from build123d import *

# Parameters (mm, degrees)
SKETCH_1_R          = 7
EXTRUDE_1_DEPTH     = 1
SKETCH_2_R          = 5
EXTRUDE_2_DEPTH     = 6
EXTRUDE_START       = 11
SKETCH_3_R          = 7
EXTRUDE_3_DEPTH     = 11
SKETCH_4_R          = 4
CUT_EXTRUDE_1_DEPTH = 21.542638584


with BuildPart() as part:
    # Эскиз1 → Бобышка-Вытянуть1 (new body)
    with BuildSketch(Plane.XY):
        Circle(SKETCH_1_R)
    extrude(amount=EXTRUDE_1_DEPTH)

    # Эскиз2 → Бобышка-Вытянуть2 (add)
    with BuildSketch(Plane(origin=(0, 0, 0), x_dir=(-1, 0, 0), z_dir=(0, 0, -1))):
        with Locations(Location((0, 0, 0), (0, 0, 180))):
            Circle(SKETCH_2_R)
    extrude(amount=EXTRUDE_2_DEPTH)

    # Эскиз3 → Бобышка-Вытянуть3 (add)
    with BuildSketch(Plane(origin=(0, 0, -6), x_dir=(-1, 0, 0), z_dir=(0, 0, -1)).offset(EXTRUDE_START)):
        with Locations(Location((0, 0, 0), (0, 0, 180))):
            Circle(SKETCH_3_R)
    extrude(amount=-EXTRUDE_3_DEPTH)

    # Эскиз4 → Вырез-Вытянуть1 (cut, through all)
    with BuildSketch(Plane(origin=(0, 0, -17), x_dir=(-1, 0, 0), z_dir=(0, 0, -1))):
        Circle(SKETCH_4_R)
    extrude(amount=-CUT_EXTRUDE_1_DEPTH, mode=Mode.SUBTRACT)


solid = part.part
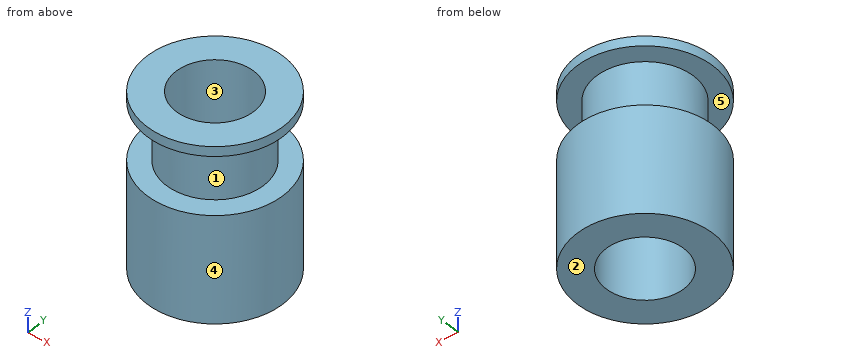
Verification items for the finished model (mm, model axes). Face numbers are marked on the shaded views. A direction names the side the tool comes from. Round coordinates to 2 decimals unless told otherwise and drop trailing zeros. Write each loop counter-clockwise with the first axis right and the second up, starting at its lowest first coordinate (ties: lowest second). Pieces come first, ordered by that corner, then holes.
(1) Mould release check, pull along Y, two halves, no side actions. Record for the marked faces 3, 4 and 5: pulls with the +Y half, pulls with the -Y half, needs draft (parallel to the pull), parting line crosses it, or undercut.
Returned:
face 3: undercut
face 4: parting line crosses it
face 5: needs draft
(2) Depth check by flat-ended pin: pin 1 Ø1 at (y, z) = (1, -4.5) entering from -X; pin 2 Ø4 at (x, z) = (4.5, -10.5) entering from +Y; pin 3 Ø8 at (x, z) = (-5.5, -9.5) entering from -Y. Enter the tip coordinate at first touch or a pass-through.
Returned:
pin 1: stops at x = -4.97
pin 2: stops at y = 6.54
pin 3: stops at y = -6.84
(3) Section check D-D (z = -9.25). Enter the section's corners in (x, y), plus the area to 3 significant figures.
Returned:
outline: circle Ø14 at (0, 0); hole circle Ø8 at (0, 0)
area: 104 mm2
(4) Material ranges on line 1 (Z direction, x = -5.5, y = 0.25); line 2 (Y direction, x = 0, z = -13.5); line 3 (Y direction, x = 0, z = -2.75), recorded low to high.
Returned:
line 1: z = -17 to -6, 0 to 1
line 2: y = -7 to -4, 4 to 7
line 3: y = -5 to -4, 4 to 5
(5) Access from +Z, -Z, +X, -X, +Y, -Y to the whole of each face (thin tool, end or side, straight path). Record for the marked faces 1 and 2.
Returned:
face 1: none
face 2: -Z, +X, -X, +Y, -Y
(6) Section check C-C (z = -3.75). Enter the section's corners in (x, y).
Returned:
outline: circle Ø10 at (0, 0); hole circle Ø8 at (0, 0)
(7) Section check A-A (y = 0). Enter the section's corners in (x, z), plus the area to 3 significant figures.
Returned:
outline: (-7, -17) - (-4, -17) - (-4, 1) - (-7, 1) - (-7, 0) - (-5, 0) - (-5, -6) - (-7, -6) - close; (4, -17) - (7, -17) - (7, -6) - (5, -6) - (5, 0) - (7, 0) - (7, 1) - (4, 1) - close
area: 84.0 mm2
